from build123d import *

# Parameters (mm, degrees)
BOSS_EXTRUDE1_DEPTH = 8
SKETCH3_R           = 10.068967795
BOSS_EXTRUDE2_DEPTH = 63
CUT_EXTRUDE1_DEPTH  = 83
SKETCH7_R           = 1.5
CUT_EXTRUDE2_DEPTH  = 10
SKETCH9_W           = 23.5
SKETCH9_H           = 2
CUT_EXTRUDE3_DEPTH  = 8
SKETCH10_W          = 12.086915154
SKETCH10_H          = 22.82391002
CUT_EXTRUDE4_DEPTH  = 48
CUT_EXTRUDE5_DEPTH  = 14


with BuildPart() as part:
    # Sketch2 → Boss-Extrude1 (new body)
    with BuildSketch(Plane.XY):
        Polygon((0, 0), (38, 0), (38, -9), (29.068967795, -18.918916137), (29.068967795, -20.918916137), (8.931032205, -20.918916137), (8.931032205, -18.918916137), (0, -9), align=None)
    extrude(amount=BOSS_EXTRUDE1_DEPTH)

    # Sketch3 → Boss-Extrude2 (add)
    with BuildSketch(Plane.XZ.offset(20.918916137)):
        with Locations((19, 4)):
            Circle(SKETCH3_R)
    extrude(amount=BOSS_EXTRUDE2_DEPTH)

    # Sketch4 → Cut-Extrude1 (cut)
    with BuildSketch(Plane(origin=(0, 0, 0), x_dir=(0, 0, -1), z_dir=(1, 0, 0))):
        Polygon((0, -20.918916137), (6.068967795, -31.271096096), (6.068967795, -20.918916137), align=None)
        Polygon((-14.068967795, -20.918916137), (-8, -20.918916137), (-14.068967795, -31.271096096), align=None)
    extrude(amount=CUT_EXTRUDE1_DEPTH, mode=Mode.SUBTRACT)

    # Sketch7 → Cut-Extrude2 (cut)
    with BuildSketch(Plane(origin=(0, 0, 0), x_dir=(-1, 0, 0), z_dir=(0, 0, -1))):
        with Locations((-22, -3)):
            Circle(SKETCH7_R)
        with Locations((-16, -3)):
            Circle(SKETCH7_R)
    extrude(amount=-CUT_EXTRUDE2_DEPTH, mode=Mode.SUBTRACT)

    # Sketch9 → Cut-Extrude3 (cut)
    with BuildSketch(Plane(origin=(0, 0, 0), x_dir=(1, 0, 0), z_dir=(0, 1, 0))):
        with Locations((19, -4)):
            Rectangle(SKETCH9_W, SKETCH9_H)
    extrude(amount=-CUT_EXTRUDE3_DEPTH, mode=Mode.SUBTRACT)

    # Sketch10 → Cut-Extrude4 (cut)
    with BuildSketch(Plane(origin=(0, 0, 0), x_dir=(0, 0, -1), z_dir=(1, 0, 0))):
        with Locations((0.025510218, -69.006961127)):
            Rectangle(SKETCH10_W, SKETCH10_H)
    extrude(amount=CUT_EXTRUDE4_DEPTH, mode=Mode.SUBTRACT)

    # Sketch12 → Cut-Extrude5 (cut)
    with BuildSketch(Plane.XZ.offset(83.918916137)):
        with BuildLine():
            Line((12.623924181, 4.142800634), (25.864458584, 4.142800634))
            ThreePointArc((25.864458584, 4.142800634), (27.364458584, 2.642800634), (25.864458584, 1.142800634))
            Line((25.864458584, 1.142800634), (12.623924181, 1.142800634))
            ThreePointArc((12.623924181, 1.142800634), (11.123924181, 2.642800634), (12.623924181, 4.142800634))
        make_face()
    extrude(amount=-CUT_EXTRUDE5_DEPTH, mode=Mode.SUBTRACT)


solid = part.part
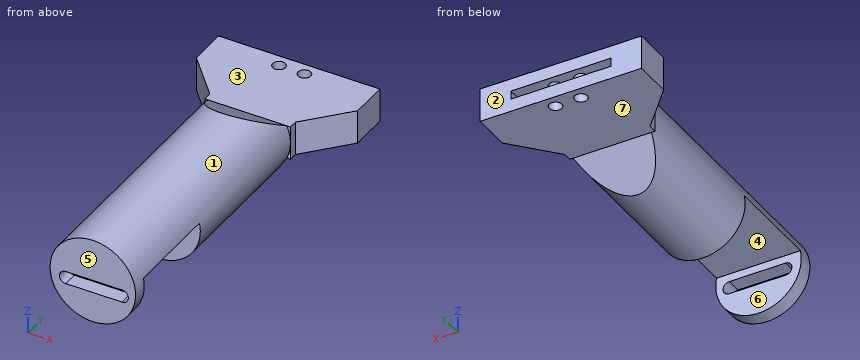
Verification items for the finished model (mm, model axes). Face numbers are marked on the shaded views. A direction names the side the tool comes from. Give positions to 0.01 mm unless a question says otherwise; leave off trailing zeros. Loops run counter-clockwise (first coordinate to the right, second up) from the corner with the lowest first, then second, coordinate; pieces in that order, holes last. Notation, with made-up numbers: (7.25, 61.25) - (22.25, 61.25) arc R30 ccw to (22.25, 97.25) - close; hole circle Ø10 at (68, -17.5). An arc over 180 degrees is marked (long way). Write item = value, one per line. Start each with the question number.
Q1. Cross-section at A-A, the plane y = -3. Enter the section's corners in (x, z), and give its area (3 significant figures).
Q2. Depth check by flat-ended pin: P1, Ø10, axis at y = -33, z = -3.5, coming from the +X side; P2, Ø5, axis at x = 15, y = -13, coming from the +Z side; P3, Ø10.5, axis at x = 19.5, y = -11, coming from the -Z side; P4, Ø2.5, axis at x = 16, y = -3, coming from the -Z side. Enter the tip coordinate at first touch or a pass-through.
Q3. Cross-section at C-C, the plane z = -3. Enter the section's corners in (x, y) (3 decimals).
Q4. Cross-section at B-B, the plane x = 19. Enter the section's corners in (y, z) (3 decimals), and give its area (3 significant figures).
Q5. Cross-section at D-D, the plane y = -35. Enter the section's corners in (x, z), and give its area (3 significant figures).
Q6. Mould release check, pull along Y, two halves, no side actions. Record for the marked faces 4, 5, 6 and 7: released by +Y, released by -Y, zero draft, split by the parting line, or undercut.
Q7. Tool access check on the marked faces 1, 2 and 3. Record the directions out of +Z, -Z, +X, -X, +Y, -Y that give a thin tool (end or side, any length) a straight path to the whole face; none if there is none.
Q8. Thickness scan on line 1 (Y direction, x = 16, z = 7.45); line 2 (Z direction, x = 20, y = -4); line 3 (Y direction, x = 22, z = 2.45) (3 decimals). Record the ranges inside material, lowest first.
Answer key:
q1.outline = (0, 0) - (14.5, 0) - (14.5, 3) - (7.25, 3) - (7.25, 5) - (14.5, 5) - (14.5, 8) - (0, 8) - close; (17.5, 0) - (20.5, 0) - (20.5, 3) - (17.5, 3) - close; (17.5, 5) - (20.5, 5) - (20.5, 8) - (17.5, 8) - close; (23.5, 0) - (38, 0) - (38, 8) - (23.5, 8) - (23.5, 5) - (30.75, 5) - (30.75, 3) - (23.5, 3) - close
q1.area = 221 mm^2
q2.P1 = 28.75
q2.P2 = 8
q2.P3 = 0
q2.P4 = through
q3.outline = (11.762, -83.919) - (26.238, -83.919) - (26.238, -80.419) - (11.762, -80.419) - close; (11.762, -57.595) - (26.238, -57.595) - (26.238, -26.036) - (11.762, -26.036) - close
q4.outline = (-83.919, -6.069) - (-80.419, -6.069) - (-80.419, 1.143) - (-83.919, 1.143) - close; (-83.919, 4.143) - (-80.419, 4.143) - (-80.419, 6.018) - (-57.595, 6.018) - (-57.595, -6.069) - (-31.271, -6.069) - (-20.919, 0) - (0, 0) - (0, 3) - (-8, 3) - (-8, 5) - (0, 5) - (0, 8) - (-20.919, 8) - (-31.271, 14.069) - (-83.919, 14.069) - close
q4.area = 1,070 mm^2
q5.outline = circle Ø20.14 at (19, 4)
q5.area = 319 mm^2
q6.face_4 = undercut
q6.face_5 = released by -Y
q6.face_6 = undercut
q6.face_7 = zero draft
q7.face_1 = -Y
q7.face_2 = +Z, -Z, +X, -X, +Y
q7.face_3 = +Z, +X, -X, +Y
q8.line_1 = -83.92 to -4.5, -1.5 to 0
q8.line_2 = 0 to 3, 5 to 8
q8.line_3 = -57.595 to -4.5, -1.5 to 0
